Geometry check sheet. Reference: drawing and pictorial views, mm from the part's lowest x, y, z. A direction names the side the tool comes from. Coordinates: 2 decimals unless noted, no trailing zeros. Loops run counter-clockwise (first coordinate to the right, second up) from the corner with the lowest first, then second, coordinate; pieces in that order, holes last. Notation, with made-up numbers: (-7, 14) -> (43, 14) arc R15 ccw to (43, 35) -> close; hole circle Ø7 at (-1, 57). An arc over 180 degrees is marked (long way). Answer as a JSON object with one key per item and string values.
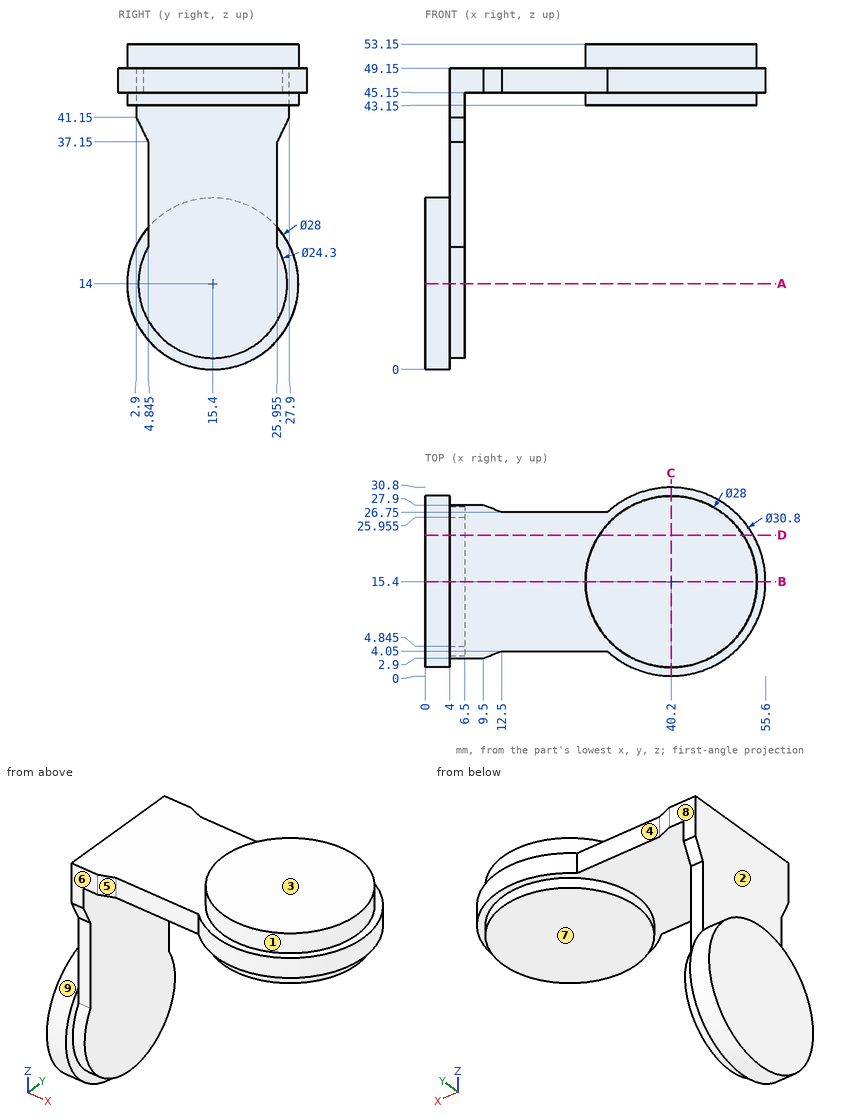
1. Tool access check on the marked faces 5, 6, 7, 8 and 9. Record the directions out of +Z, -Z, +X, -X, +Y, -Y that give a thin tool (end or side, any length) a straight path to the whole face; none if there is none.
Evaluation:
{"face 5": "+Z, -Z, -Y", "face 6": "+Z, -Z, -X, -Y", "face 7": "-Z, +X, +Y, -Y", "face 8": "+Z, -Z, -X, +Y", "face 9": "-X"}
2. Mould release check, pull along X, two halves, no side actions. Record for the marked faces 1, 2, 3 and 4: released by +X, released by -X, zero draft, split by the parting line, or undercut.
Evaluation:
{"face 1": "split by the parting line", "face 2": "released by -X", "face 3": "zero draft", "face 4": "undercut"}
3. Section check C-C, the plane x = 40.2. Record the boundary of the cut face in (y, z), then the cut area to 3 significant figures.
Evaluation:
{"outline": "(0, 45.15) -> (1.4, 45.15) -> (1.4, 43.15) -> (29.4, 43.15) -> (29.4, 45.15) -> (30.8, 45.15) -> (30.8, 49.15) -> (29.4, 49.15) -> (29.4, 53.15) -> (1.4, 53.15) -> (1.4, 49.15) -> (0, 49.15) -> close", "area": "291 mm^2"}
4. Thickness scan on probe 1 along Z at (x, y) = (40.5, 20.5); probe 2 along Z at (x, y) = (23, 6.5); probe 3 along X at (y, z) = (20, 41.5). Record the ranges inside material, lowest first. Write a range as from..to.
Evaluation:
{"probe 1": "z = 43.15..53.15", "probe 2": "z = 45.15..49.15", "probe 3": "x = 4..6.5"}
5. Section check B-B, the plane y = 15.4. Record the boundary of the cut face in (x, z), then the cut area to 3 significant figures.
Evaluation:
{"outline": "(0, 0) -> (4, 0) -> (4, 1.85) -> (6.5, 1.85) -> (6.5, 45.15) -> (26.2, 45.15) -> (26.2, 43.15) -> (54.2, 43.15) -> (54.2, 45.15) -> (55.6, 45.15) -> (55.6, 49.15) -> (54.2, 49.15) -> (54.2, 53.15) -> (26.2, 53.15) -> (26.2, 49.15) -> (4, 49.15) -> (4, 28) -> (0, 28) -> close", "area": "595 mm^2"}
6. Section check A-A, the plane z = 14. Record the boundary of the cut face in (x, y).
Evaluation:
{"outline": "(0, 1.4) -> (4, 1.4) -> (4, 3.25) -> (6.5, 3.25) -> (6.5, 27.55) -> (4, 27.55) -> (4, 29.4) -> (0, 29.4) -> close"}
7. Section check D-D, the plane y = 23. Record the boundary of the cut face in (x, z).
Evaluation:
{"outline": "(0, 2.24) -> (4, 2.24) -> (4, 4.52) -> (6.5, 4.52) -> (6.5, 45.15) -> (28.44, 45.15) -> (28.44, 43.15) -> (51.96, 43.15) -> (51.96, 45.15) -> (53.59, 45.15) -> (53.59, 49.15) -> (51.96, 49.15) -> (51.96, 53.15) -> (28.44, 53.15) -> (28.44, 49.15) -> (4, 49.15) -> (4, 25.76) -> (0, 25.76) -> close"}
8. Depth check by flat-ended pin: P1, Ø1, axis at x = 49, z = 43, coming from the -Y side; P2, Ø12.5, axis at y = 18.5, z = 22.5, coming from the +X side; P3, Ø3, axis at x = 5, z = 27, coming from the -Y side (1 decimal). Enter the tip coordinate at first touch or a pass-through.
Evaluation:
{"P1": "stops at y = 4.14", "P2": "stops at x = 6.5", "P3": "stops at y = 4.8"}
